from build123d import *

# Parameters (mm, degrees)
ESQUISSE1_W             = 10
ESQUISSE1_H             = 6
BOSS_EXTRU_1_DEPTH      = 6
ESQUISSE2_R             = 12.5
ESQUISSE2_R_2           = 7.5
ESQUISSE2_R_3           = 5
ENL_V_MAT_EXTRU_1_DEPTH = 6
CONG_1_R                = 10


with BuildPart() as part:
    # Esquisse1 → Boss.-Extru.1 (new body)
    # profile 1 of 2: a face of its own
    with BuildSketch(Plane(origin=(0, 0, 0), x_dir=(1, 0, 0), z_dir=(0, 1, 0))):
        Polygon((0, 359), (0, 185), (67, 185), (67, 370), (25.728690358, 370), (25.728690358, 359), align=None)
        with Locations((44, 362)):
            Rectangle(ESQUISSE1_W, ESQUISSE1_H, mode=Mode.SUBTRACT)
    # profile 2 of 2: a face of its own
    with BuildSketch(Plane(origin=(0, 0, 0), x_dir=(1, 0, 0), z_dir=(0, 1, 0))):
        Polygon((67, 185), (0, 185), (0, 11), (25.728690358, 11), (25.728690358, 0), (67, 0), align=None)
        with Locations((44, 8)):
            Rectangle(ESQUISSE1_W, ESQUISSE1_H, mode=Mode.SUBTRACT)
    extrude(amount=BOSS_EXTRU_1_DEPTH)

    # Esquisse2 → Enlèv. mat.-Extru.1 (cut)
    with BuildSketch(Plane(origin=(0, 6, 0), x_dir=(1, 0, 0), z_dir=(0, 1, 0))):
        with Locations(Location((51, 338, 0), (0, 0, 270))):
            Circle(ESQUISSE2_R)
        with Locations(Location((51, 304, 0), (0, 0, 270))):
            Circle(ESQUISSE2_R)
        with Locations(Location((51, 270, 0), (0, 0, 270))):
            Circle(ESQUISSE2_R)
        with Locations(Location((51, 236, 0), (0, 0, 270))):
            Circle(ESQUISSE2_R)
        with Locations(Location((51, 202, 0), (0, 0, 270))):
            Circle(ESQUISSE2_R)
        with Locations(Location((51, 168, 0), (0, 0, 270))):
            Circle(ESQUISSE2_R)
        with Locations(Location((51, 134, 0), (0, 0, 270))):
            Circle(ESQUISSE2_R)
        with Locations(Location((51, 100, 0), (0, 0, 270))):
            Circle(ESQUISSE2_R)
        with Locations(Location((51, 66, 0), (0, 0, 270))):
            Circle(ESQUISSE2_R)
        with Locations(Location((26, 338, 0), (0, 0, 270))):
            Circle(ESQUISSE2_R_2)
        with Locations(Location((8, 338, 0), (0, 0, 270))):
            Circle(ESQUISSE2_R_3)
        with Locations(Location((26, 304, 0), (0, 0, 270))):
            Circle(ESQUISSE2_R_2)
        with Locations(Location((8, 304, 0), (0, 0, 270))):
            Circle(ESQUISSE2_R_3)
        with Locations(Location((26, 270, 0), (0, 0, 270))):
            Circle(ESQUISSE2_R_2)
        with Locations(Location((8, 270, 0), (0, 0, 270))):
            Circle(ESQUISSE2_R_3)
        with Locations(Location((26, 236, 0), (0, 0, 270))):
            Circle(ESQUISSE2_R_2)
        with Locations(Location((8, 236, 0), (0, 0, 270))):
            Circle(ESQUISSE2_R_3)
        with Locations(Location((26, 202, 0), (0, 0, 270))):
            Circle(ESQUISSE2_R_2)
        with Locations(Location((8, 202, 0), (0, 0, 270))):
            Circle(ESQUISSE2_R_3)
        with Locations(Location((26, 168, 0), (0, 0, 270))):
            Circle(ESQUISSE2_R_2)
        with Locations(Location((8, 168, 0), (0, 0, 270))):
            Circle(ESQUISSE2_R_3)
        with Locations(Location((26, 134, 0), (0, 0, 270))):
            Circle(ESQUISSE2_R_2)
        with Locations(Location((8, 134, 0), (0, 0, 270))):
            Circle(ESQUISSE2_R_3)
        with Locations(Location((26, 100, 0), (0, 0, 270))):
            Circle(ESQUISSE2_R_2)
        with Locations(Location((8, 100, 0), (0, 0, 270))):
            Circle(ESQUISSE2_R_3)
        with Locations(Location((26, 66, 0), (0, 0, 270))):
            Circle(ESQUISSE2_R_2)
        with Locations(Location((8, 66, 0), (0, 0, 270))):
            Circle(ESQUISSE2_R_3)
        with Locations(Location((26, 32, 0), (0, 0, 270))):
            Circle(ESQUISSE2_R_2)
        with Locations(Location((8, 32, 0), (0, 0, 270))):
            Circle(ESQUISSE2_R_3)
        with Locations(Location((51, 32, 0), (0, 0, 270))):
            Circle(ESQUISSE2_R)
    extrude(amount=-ENL_V_MAT_EXTRU_1_DEPTH, mode=Mode.SUBTRACT)

    # Congé1
    cong_1_edges = [part.edges().sort_by_distance(p)[0] for p in [
        (67, 3, -370),
        (67, 3, 0),
    ]]
    fillet(cong_1_edges, radius=CONG_1_R)


solid = part.part
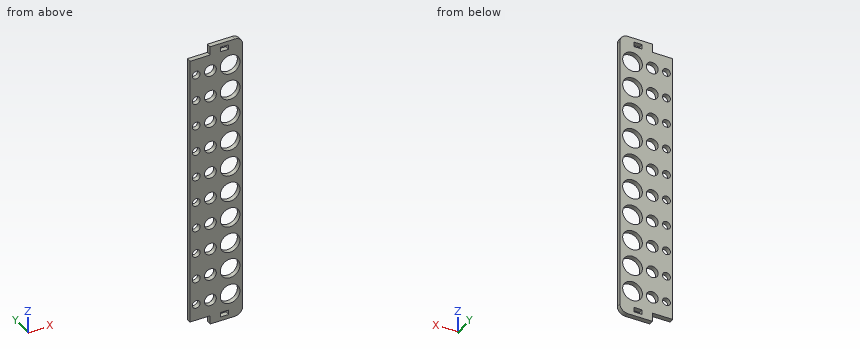
Could you check a few things on this model? Use its own coordinates, in mm. Round coordinates to 2 decimals unless told otherwise and drop trailing zeros. Loops run counter-clockwise (first coordinate to the right, second up) from the corner with the lowest first, then second, coordinate; pieces in that order, holes last. Notation, with made-up numbers: (39, 28) - (98, 28) arc R24 ccw to (98, 55) - close; hole circle Ø3 at (74.25, 7). An arc over 180 degrees is marked (long way). Write item = value, one per line.
1) Imagine slicing it at A-A (z = -66). Please give me the cut outline in (x, y).
Computed:
outline = (0, 0) - (3, 0) - (3, 6) - (0, 6) - close; (13, 0) - (18.5, 0) - (18.5, 6) - (13, 6) - close; (33.5, 0) - (38.5, 0) - (38.5, 6) - (33.5, 6) - close; (63.5, 0) - (67, 0) - (67, 6) - (63.5, 6) - close
2) Imagine slicing it at B-B (x = 8). Give the number of separate pieces and of enclosed holes in the cut face, and give its area (3 significant figures).
Computed:
separate_pieces = 11
enclosed_holes = 0
area = 1,490 mm2
3) I'm going to push a flat-ended pin straight in: P1, Ø1.8, axis at y = 1.5, z = -360.5, coming from the -X side. Where does the tip first touch, or does it pass through?
Computed:
P1 = 25.73
4) I need wall thicknesses on line 1 along X through (y, z) = (4.75, -134.5); line 2 along X through (y, z) = (4.3, -137.5). Which ranges of each line are inside material? Lowest first, please. Write a range as from..to.
Computed:
line_1 = 0..3.03, 12.97..18.52, 33.48..38.51, 63.49..67
line_2 = 0..4.43, 11.57..19.37, 32.63..39, 63..67
